from build123d import *

# Parameters (mm, degrees)
SKETCH2_W          = 7
SKETCH2_H          = 1.2
CUT_EXTRUDE1_DEPTH = 1.2


with BuildPart() as part:
    # Sketch1 → Revolve1 (revolve)
    with BuildSketch(Plane.XY):
        Polygon((0, 0), (0, 3.5), (2.6, 3.5), (2.6, 2), (8.6, 2), (8.6, 0), align=None)
    revolve(axis=Axis((8.6, 0, 0), (-1, 0, 0)))

    # Sketch2 → Cut-Extrude1 (cut)
    with BuildSketch(Plane.ZY):
        Rectangle(SKETCH2_W, SKETCH2_H)
    extrude(amount=-CUT_EXTRUDE1_DEPTH, mode=Mode.SUBTRACT)


solid = part.part
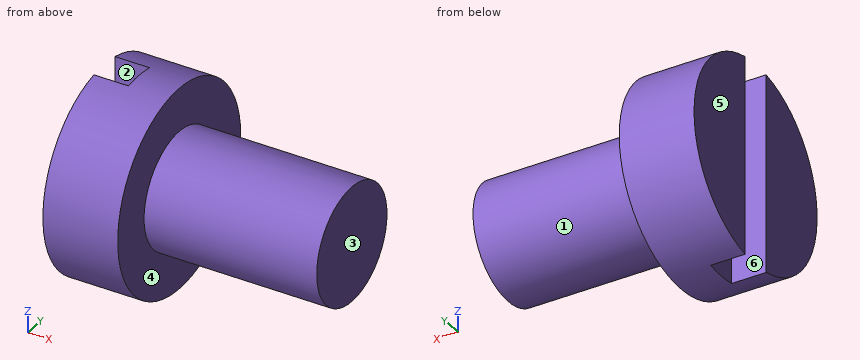
Input: part model. Units: mm. Frame: model coordinates. Face numbers are marked on the shaded views. A direction names the side the tool comes from. Give positions to 0.01 mm unless a question says otherwise; leave off trailing zeros. Loops run counter-clockwise (first coordinate to the right, second up) from the corner with the lowest first, then second, coordinate; pieces in that order, holes last. Notation, with made-up numbers: (11.25, 3.25) -> (57.25, 3.25) arc R15 ccw to (57.25, 12.25) -> close; hole circle Ø3 at (-32, -4.75). An arc over 180 degrees is marked (long way). Answer as a JSON object with one key per item and string values. Group by question number.
Item 1: Reachability of the marked faces 4, 5 and 6 from +Z, -Z, +X, -X, +Y, -Y: full face, straight path, thin tool, end or side. Return the list, or none.
Item 2: Cut plane C-C, the plane z = 0. Return the cut outline in (x, y).
Item 3: Pin query (flat end, axial travel): P1, Ø0.6, axis at x = 0.5, z = 1.5, coming from the +Y side; P2, Ø4, axis at x = 5.5, z = 1, coming from the -Y side; P3, Ø0.6, axis at y = 0, z = 1.5, coming from the -X side. Return the tip coordinate at first contact, or that it passes through.
Item 4: Cut plane D-D, the plane x = 4.25. Return the cut outline in (y, z), and give its area (3 significant figures).
Item 5: Cut plane B-B, the plane x = 1. Return the cut outline in (y, z).
Item 6: Line query: probe 1 along X at (y, z) = (3, 1); probe 2 along Y at (x, z) = (0.75, -1.25); probe 3 along Y at (x, z) = (6.5, 0). Output: solid intervals per line, ascending.
Item 7: Cut plane A-A, the plane y = 0. Return the cut outline in (x, z), and give its area (3 significant figures).
Item 8: Pull-direction query (Y, two-part tool) for the marked faces 1, 2 and 3; classes: released by +Y, released by -Y, zero draft, split by the parting line, or undercut.
Checks:
{
 "1": {"face 4": "+X", "face 5": "+Z, -Z, -X, +Y, -Y", "face 6": "+Z, -Z, -X"},
 "2": {"outline": "(0, -3.5) -> (2.6, -3.5) -> (2.6, -2) -> (8.6, -2) -> (8.6, 2) -> (2.6, 2) -> (2.6, 3.5) -> (0, 3.5) -> (0, 0.6) -> (1.2, 0.6) -> (1.2, -0.6) -> (0, -0.6) -> close"},
 "3": {"P1": "stops at y = 3.29", "P2": "stops at y = -2", "P3": "stops at x = 1.2"},
 "4": {"outline": "circle Ø4 at (0, 0)", "area": "12.6 mm²"},
 "5": {"outline": "(-0.6, -3.45) -> (-0.6, 3.45) arc R3.5 ccw to start; (0.6, -3.45) arc R3.5 ccw to (0.6, 3.45) -> close"},
 "6": {"probe 1": "x = 0 to 2.6", "probe 2": "y = -3.27 to -0.6, 0.6 to 3.27", "probe 3": "y = -2 to 2"},
 "7": {"outline": "(1.2, -3.5) -> (2.6, -3.5) -> (2.6, -2) -> (8.6, -2) -> (8.6, 2) -> (2.6, 2) -> (2.6, 3.5) -> (1.2, 3.5) -> close", "area": "33.8 mm²"},
 "8": {"face 1": "split by the parting line", "face 2": "undercut", "face 3": "zero draft"}
}
